Geometry check sheet. Reference: drawing and pictorial views, mm from the part's lowest x, y, z. A direction names the side the tool comes from. Round coordinates to 2 decimals unless told otherwise and drop trailing zeros. Loops run counter-clockwise (first coordinate to the right, second up) from the corner with the lowest first, then second, coordinate; pieces in that order, holes last. Notation, with made-up numbers: (-4.5, 50.25) -> (39.5, 50.25) arc R29 ccw to (39.5, 76.25) -> close; hole circle Ø1 at (63, 4). An arc over 180 degrees is marked (long way). Write item = value, one per line.
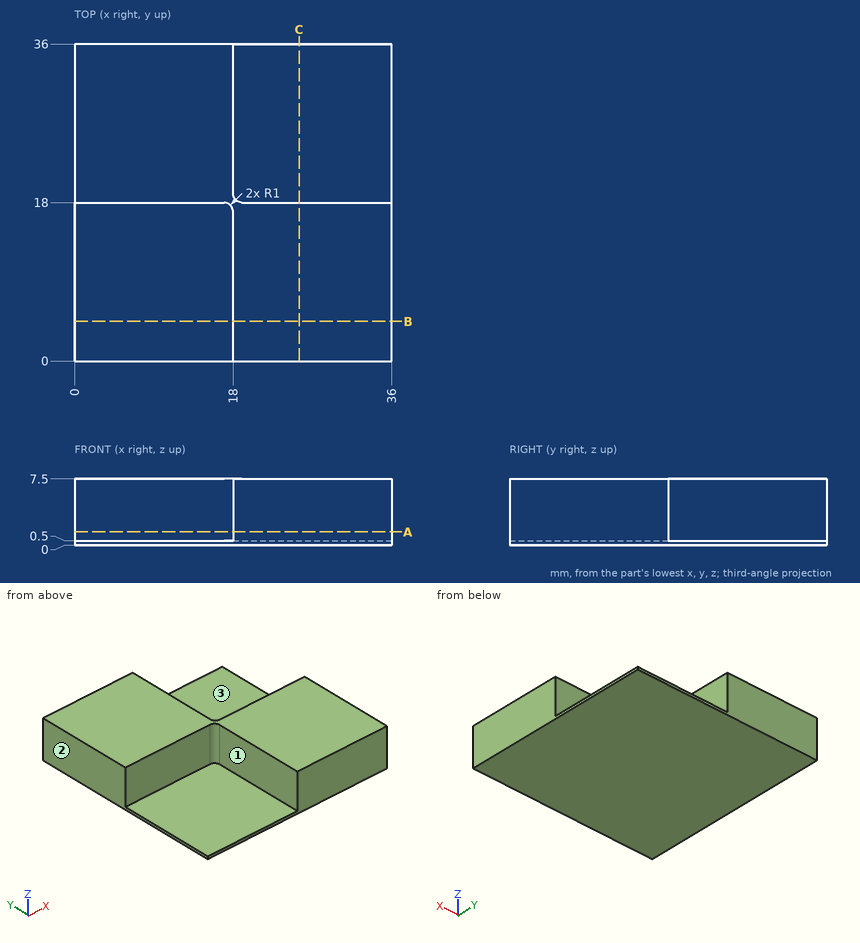
(1) Sectioned sample at C-C, the plane x = 25.5. Record the cut outline in (y, z).
Filled sheet:
outline = (0, 0) -> (36, 0) -> (36, 0.5) -> (18, 0.5) -> (18, 7.5) -> (0, 7.5) -> close
(2) Set-up check for the marked faces 1, 2 and 3: record each of +Z, -Z, +X, -X, +Y, -Y from which the full face is reachable in a straight line by a thin tool's end or side.
Filled sheet:
face_1 = +Z, -X, -Y
face_2 = +Z, -Z, -X, +Y, -Y
face_3 = +Z, +X, +Y
(3) Material ranges on probe 1 along X at (y, z) = (2.5, 5.5); probe 2 along X at (y, z) = (28, 3.5); probe 3 along Z at (x, y) = (16.5, 2), recorded low to high. Write a range as from..to.
Filled sheet:
probe_1 = 18..36
probe_2 = 0..18
probe_3 = 0..0.5
(4) Sectioned sample at A-A, the plane z = 1.5. Record the cut outline in (x, y).
Filled sheet:
outline = (0, 18) -> (17, 18) arc R1 cw to (18, 17) -> (18, 0) -> (36, 0) -> (36, 18) -> (19, 18) arc R1 cw to (18, 19) -> (18, 36) -> (0, 36) -> close
(5) Sectioned sample at B-B, the plane y = 4.5. Record the cut outline in (x, z), and give its area (3 significant figures).
Filled sheet:
outline = (0, 0) -> (36, 0) -> (36, 7.5) -> (18, 7.5) -> (18, 0.5) -> (0, 0.5) -> close
area = 144 mm2
(6) Go/stop test with flat-tipped pins: pin 1 Ø2 at (y, z) = (7, 3) entering from -X; pin 2 Ø2 at (x, z) = (19.5, 6) entering from +Y; pin 3 Ø2 at (x, z) = (10.5, 4.5) entering from -Y. Record where each tip stops, or that it passes through.
Filled sheet:
pin_1 = 18
pin_2 = 18.13
pin_3 = 18
